Verification items for the finished model (mm, model axes). Coordinates: 2 decimals unless noted, no trailing zeros. Order: outer loops, then holes, each group sorted by start corner. A loop starts at its lowest first (then second) coordinate and runs counter-clockwise, first axis right, second up. Notation, with made-up numbers: M 66,-10.5 L 74,-10.5 A20 cw 74,9.5 Z; hole C 65,27 d3. An arc over 180 degrees is marked long. Write item = value, one per line.
```python
from build123d import *

# Parameters (mm, degrees)
ESQUISSE1_R        = 6.45
ESQUISSE1_R_2      = 5.15
BOSS_EXTRU_1_DEPTH = 4.7
BOSS_EXTRU_1_DRAFT = 2
ESQUISSE2_R        = 6.285872383
ESQUISSE2_R_2      = 2.65
BOSS_EXTRU_2_DEPTH = 1
CONG_1_R           = 0.5


with BuildPart() as part:
    # Esquisse1 → Boss.-Extru.1 (with draft: the straight prism first)
    with BuildSketch(Plane.XY):
        Circle(ESQUISSE1_R)
        Circle(ESQUISSE1_R_2, mode=Mode.SUBTRACT)
    extrude(amount=BOSS_EXTRU_1_DEPTH)
    # Boss.-Extru.1: the draft: its side faces are tilted about the plane it starts from
    boss_extru_1_sides = [part.faces().sort_by_distance(p)[0] for p in [
        (-6.45, 0, 2.35),
        (-5.15, 0, 2.35),
    ]]
    draft(boss_extru_1_sides, Plane.XY, BOSS_EXTRU_1_DRAFT)

    # Esquisse2 → Boss.-Extru.2 (add)
    with BuildSketch(Plane.XY.offset(4.7)):
        Circle(ESQUISSE2_R)
        Circle(ESQUISSE2_R_2, mode=Mode.SUBTRACT)
    extrude(amount=-BOSS_EXTRU_2_DEPTH)

    # Congé1
    cong_1_edges = [part.edges().sort_by_distance(p)[0] for p in [
        (-6.285872383, 0, 4.7),
    ]]
    fillet(cong_1_edges, radius=CONG_1_R)


solid = part.part
```
Item 1: Sectioned sample at C-C, the plane z = 0.5. Enter the section's corners in (x, y).
Report:
outline = C 0,0 d12.87; hole C 0,0 d10.33
Item 2: Release check for a two-part mould opening along Z. For faces 1 (the cylindrical face through (2.45, -1.01, 4.21)), 2 (the conical face through (-1.13, -5.09, 1.82)), 3 (the conical face through (-5.06, -3.88, 2.08)) record: pulls with the +Z half, pulls with the -Z half, needs draft (parallel to the pull), parting line crosses it, or undercut.
Report:
face_1 = needs draft
face_2 = undercut
face_3 = pulls with the +Z half
Item 3: Sectioned sample at D-D, the plane z = 3.5. Enter the section's corners in (x, y), then the cut area to 3 significant figures.
Report:
outline = C 0,0 d12.66; hole C 0,0 d10.54
area = 38.5 mm^2
Item 4: Sectioned sample at A-A, the plane x = 0. Enter the section's corners in (y, z), then the cut area to 3 significant figures.
Report:
outline = M -6.45,0 L -5.15,0 L -5.28,3.7 L -2.65,3.7 L -2.65,4.7 L -5.8,4.7 A0.5 ccw -6.3,4.22 Z; M 2.65,3.7 L 5.28,3.7 L 5.15,0 L 6.45,0 L 6.3,4.22 A0.5 ccw 5.8,4.7 L 2.65,4.7 Z
area = 15.9 mm^2
Item 5: Gauge pin test, flat ends, axial feed: pin 1 (1 mm diameter, centred on y = -2.5, z = 1, fed in from -X); pin 2 (2 mm diameter, centred on x = 2, z = 3, fed in from +Y); pin 3 (4 mm diameter, centred on x = 1, y = -1, fed in from +Z); pin 4 (4 mm diameter, centred on x = 0, y = 0, fed in from -Z). Record the tip position at first contact, or that the pin passes through.
Report:
pin_1 = -6.1
pin_2 = 6.27
pin_3 = 4.7
pin_4 = through
Item 6: Scan lines: L1, parallel to Z at x = -3.75, y = -1; L2, parallel to X at y = 1.5, z = 2.2; L3, parallel to Y at x = 3.5, z = 0.8. Record each from-to range of solid material in increasing order. Write a range as from..to.
Report:
L1 = 3.7..4.7
L2 = -6.19..-5.01, 5.01..6.19
L3 = -5.38..-3.82, 3.82..5.38
